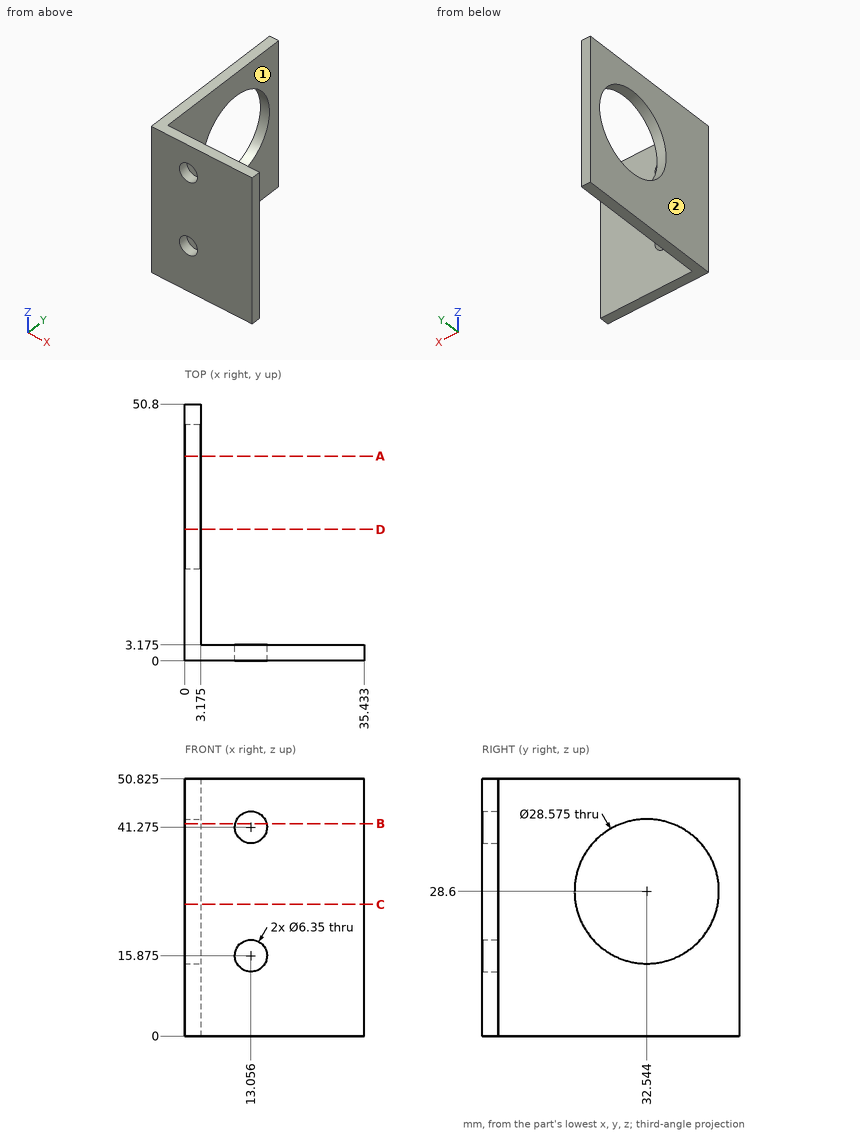
The drawing under review shows one solid part. Ordinate dimensions are in mm from its lowest x, y, z. A direction names the side the tool comes from. Coordinates: 2 decimals unless noted, no trailing zeros. Write each loop counter-clockwise with the first axis right and the second up, starting at its lowest first coordinate (ties: lowest second). Pieces come first, ordered by that corner, then holes.
1) Add section D-D (y = 26). Write out the cut boundary in (x, z) (1 decimal).
2) Add section A-A (y = 40.5). Write out the cut boundary in (x, z) (1 decimal).
3) Add section B-B (z = 42). Write out the cut boundary in (x, y) (1 decimal).
4) Insertion check: pin 1 (8 mm diameter, centred on y = 22, z = 14, fed in from +X) (3 decimals). The pin has a flat end and moves straight along its axis. Give the tip position at first contact, or say it passes through.
5) Add section C-C (z = 26). Write out the cut boundary in (x, y) (1 decimal).
6) Machinability: for the marked faces 1 and 2, which of the approach directions +Z, -Z, +X, -X, +Y, -Y give a long, thin tool a straight path to every point of the face, cutting with its end or side? Answer none if there is none.
7) To check wall thickness, follow L1, parallel to Y at x = 31, z = 39.5 (1 decimal); L2, parallel to X at y = 3, z = 43. State the ranges of each line that lie inside material, in increasing order.
Check result:
1. outline: (0, 0) - (3.2, 0) - (3.2, 15.9) - (0, 15.9) - close; (0, 41.3) - (3.2, 41.3) - (3.2, 50.8) - (0, 50.8) - close
2. outline: (0, 0) - (3.2, 0) - (3.2, 16.7) - (0, 16.7) - close; (0, 40.5) - (3.2, 40.5) - (3.2, 50.8) - (0, 50.8) - close
3. outline: (0, 0) - (10, 0) - (10, 3.2) - (3.2, 3.2) - (3.2, 27.6) - (0, 27.6) - close; (0, 37.5) - (3.2, 37.5) - (3.2, 50.8) - (0, 50.8) - close; (16.1, 0) - (35.4, 0) - (35.4, 3.2) - (16.1, 3.2) - close
4. pin 1: stops at x = 3.175
5. outline: (0, 0) - (35.4, 0) - (35.4, 3.2) - (3.2, 3.2) - (3.2, 18.5) - (0, 18.5) - close; (0, 46.6) - (3.2, 46.6) - (3.2, 50.8) - (0, 50.8) - close
6. face 1: +Z, -Z, +X, +Y
6. face 2: +Z, -Z, -X, +Y, -Y
7. L1: y = 0 to 3.2
7. L2: x = 0 to 10.39, 15.72 to 35.43
